Here's how the part is built. I have some questions about the finished solid (model axes, mm). Coordinates: 2 decimals unless noted, no trailing zeros. Order: outer loops, then holes, each group sorted by start corner. A loop starts at its lowest first (then second) coordinate and runs counter-clockwise, first axis right, second up.
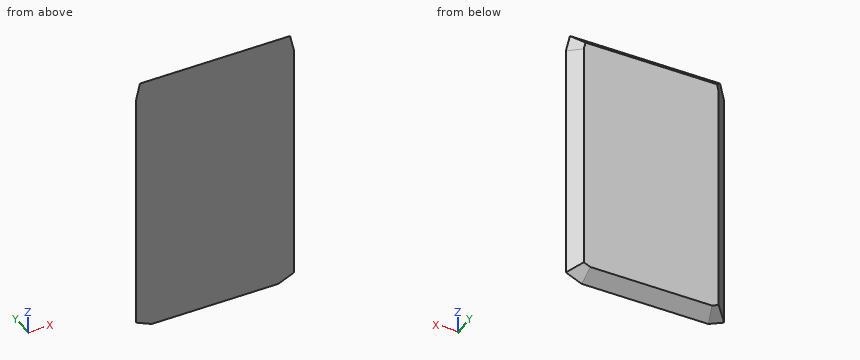
Autodesk Inventor part; units mm, degrees
ref_plane "YZ Plane" through (0, 0, 0) normal (1, 0, 0) x (0, 1, 0)
ref_plane "XZ Plane" through (0, 0, 0) normal (0, 1, 0) x (-1, 0, 0)
ref_plane "XY Plane" through (0, 0, 0) normal (0, 0, 1) x (1, 0, 0)
sketch "Sketch1" plane through (0, 0, 0) normal (0, 1, 0) x (-1, 0, 0)
  line L0 (11.1472, -12.1394) -> (32.7528, -12.1394)
  line L1 (32.7528, -12.1394) -> (11.1472, -12.1394)
  line L2 (8.45, -10.938) -> (11.1472, -12.1394)
  line L3 (11.1472, -12.1394) -> (8.45, -10.938)
  line L4 (8.45, -10.938) -> (10.45, -9.6394)
  line L5 (8.45, 30.5881) -> (8.45, -10.938)
  line L6 (8.45, -10.938) -> (8.45, 30.5881)
  line L7 (9.1529, 33.6372) -> (10.7443, 31.6372)
  line L8 (8.45, 30.5881) -> (9.1529, 33.6372)
  line L9 (35.45, -10.938) -> (35.45, 30.5881)
  line L10 (8.45, -10.938) -> (35.45, -10.938)
  line L11 (35.45, 30.5881) -> (33.45, 30.3606)
  line L12 (8.45, 30.5881) -> (35.45, 30.5881)
  line L13 (34.747, 33.6372) -> (9.1529, 33.6372)
  line L14 (9.1529, 33.6372) -> (34.747, 33.6372)
  line L15 (11.1472, -12.1394) -> (32.7528, -12.1394)
  line L16 (8.45, 30.5881) -> (9.1529, 33.6372)
  line L17 (9.1529, 33.6372) -> (34.747, 33.6372)
  line L18 (11.5725, -10.1394) -> (32.3275, -10.1394)
  line L19 (32.3275, -10.1394) -> (11.5725, -10.1394)
  line L20 (11.1472, -12.1394) -> (8.45, -10.938)
  line L21 (8.45, -10.938) -> (8.45, 30.5881)
  line L22 (8.45, 30.5881) -> (9.1529, 33.6372)
  line L23 (34.747, 33.6372) -> (9.1529, 33.6372)
  line L24 (35.45, 30.5881) -> (34.747, 33.6372)
  line L25 (34.747, 33.6372) -> (35.45, 30.5881)
  line L26 (32.7528, -12.1394) -> (35.45, -10.938)
  line L27 (32.7528, -12.1394) -> (35.45, -10.938)
  line L28 (33.45, -9.6394) -> (33.45, 30.3606)
  line L29 (32.3275, -10.1394) -> (33.45, -9.6394)
  line L30 (33.45, 30.3606) -> (33.45, -9.6394)
  line L31 (32.3275, -10.1394) -> (11.5725, -10.1394)
  line L32 (10.45, -9.6394) -> (11.5725, -10.1394)
  line L33 (11.5725, -10.1394) -> (10.45, -9.6394)
  line L34 (10.45, -9.6394) -> (10.45, 30.3606)
  line L35 (10.45, 30.3606) -> (10.7443, 31.6372)
  line L36 (33.1557, 31.6372) -> (10.7443, 31.6372)
  line L37 (33.45, 30.3606) -> (33.1557, 31.6372)
  point P0 (0, 0)
  point P1 (-34.55, -34.6394)
extrude "Extrusion1" add sketch "Sketch1" along normal blind 2
chamfer "Chamfer1" distance 2 angle 45 8 edges at (-35.45, 2, 9.8251) (-35.0985, 2, 32.1127) (-21.95, 2, 33.6372) (-8.8014, 2, 32.1127) (-8.45, 2, 9.8251) (-21.95, 2, -12.1394) (-9.7986, 2, -11.5387) (-34.1014, 2, -11.5387)
sketch "Sketch2" plane through (0, 2, 0) normal (0, 1, 0) x (1, 0, 0)
  point P0 (0, 0)
equation "\"BendRadius\" = Thickness"
equation "\"BendReliefWidth\" = Thickness"
equation "\"BendReliefDepth\" = 0.5 * Thickness"
equation "\"CornerReliefSize\" = 4 * Thickness"
equation "\"MinimumRemnant\" = 2 * Thickness"
equation "\"TransitionRadius\" = BendRadius"
equation "\"JacobiRadiusSize\" = BendRadius"
equation "\"GapSize\" = Thickness"
properties part number "Part3edd"
Q1. I need wall thicknesses on L1, parallel to Z at x = -21.75, y = 0.95; L2, parallel to Z at x = -28, y = 1.4; L3, parallel to X at y = 1.1, z = 20.5. Which ranges of each line are inside material? Lowest first, please.
Q2. If we section it at B-B on y = 0.35: Write out the boundary of the cut face in (x, z).
Q3. Will this pin go through, and if not, where does the flat tip stop? pin 1 (1 mm diameter, centred on y = 1, z = 6.5, fed in from +X).
Reply:
1. L1: z = -11.19 to 32.69
1. L2: z = -10.74 to 32.24
1. L3: x = -34.35 to -9.55
2. outline: (-35.1, -10.71) - (-32.68, -11.79) - (-11.22, -11.79) - (-8.8, -10.71) - (-8.8, 30.55) - (-9.43, 33.29) - (-34.47, 33.29) - (-35.1, 30.55) - close
3. pin 1: stops at x = -8.95
